Part model, mm, in its own coordinate system. A direction names the side the tool comes from. Round coordinates to 2 decimals unless told otherwise and drop trailing zeros. Write each loop counter-clockwise with the first axis right and the second up, starting at its lowest first coordinate (ties: lowest second). Pieces come first, ordered by that corner, then holes. Notation, with made-up numbers: (-20, -5) -> (-12, -5) arc R12 cw to (-12, 4) -> close; hole circle Ø10 at (-27, 2.5). An arc over 180 degrees is marked (long way). Return JSON: item names as keys, results as strings. Group by question number.
```python
from build123d import *

# Parameters (mm, degrees)
SKETCH1_W           = 366
SKETCH1_H           = 19
BOSS_EXTRUDE2_DEPTH = 19
SKETCH9_W           = 17
SKETCH9_H           = 17
CUT_EXTRUDE4_DEPTH  = 367.985013318
CUT_EXTRUDE6_DEPTH  = 339.005366679
SKETCH12_R          = 2
CUT_EXTRUDE7_DEPTH  = 339.005366679


with BuildPart() as part:
    # Sketch1 → Boss-Extrude2 (new body)
    with BuildSketch(Plane(origin=(0, 0, 0), x_dir=(1, 0, 0), z_dir=(0, 1, 0))):
        with Locations((-153.935643564, 9.5)):
            Rectangle(SKETCH1_W, SKETCH1_H)
    extrude(amount=BOSS_EXTRUDE2_DEPTH)

    # Sketch9 → Cut-Extrude4 (cut, through all)
    with BuildSketch(Plane(origin=(29.064356436, 0, 0), x_dir=(0, 0, -1), z_dir=(1, 0, 0))):
        with Locations((9.5, 9.5)):
            Rectangle(SKETCH9_W, SKETCH9_H)
    extrude(amount=-CUT_EXTRUDE4_DEPTH, mode=Mode.SUBTRACT)

    # Sketch11 → Cut-Extrude6 (cut, through all)
    with BuildSketch(Plane(origin=(0, 0, -19), x_dir=(-1, 0, 0), z_dir=(0, 0, -1))):
        Polygon((-29.064356436, 19), (-29.064356436, 0), (3.935643564, 0), align=None)
        Polygon((336.935643564, 19), (336.935643564, 0), (303.935643564, 0), align=None)
    extrude(amount=-CUT_EXTRUDE6_DEPTH, mode=Mode.SUBTRACT)

    # Sketch12 → Cut-Extrude7 (cut, through all)
    with BuildSketch(Plane.XY):
        with Locations((-153.935643564, 10)):
            Circle(SKETCH12_R)
    extrude(amount=-CUT_EXTRUDE7_DEPTH, mode=Mode.SUBTRACT)


solid = part.part
```
Item 1: Flat gauge pin, fed straight in: P1, Ø5, axis at y = 3, z = -8.5, coming from the +X side. Where does the tip first touch, or does it go through?
Item 2: Cut at B-B (x = -119.5). Write the cut outline in (y, z).
Item 3: Cut at A-A (z = -14.5). Write the cut outline in (x, y).
Item 4: Wall check: L1, parallel to Y at x = -9, z = -4.5; L2, parallel to Z at x = 12, y = 14; L3, parallel to Y at x = 5, z = -9.25. Give the ranges that are in metal, low to high.
Item 5: Two-plate mould, pull along Y, no slides. Class faces 1 (the face through (-156, 9, -19)), 2 (the face through (-151, 18, -9)), 3 (the face through (11.265, 8.752, -0.396)), 4 (the face through (-151, 9, -1)): released by +Y, released by -Y, zero draft, split by the parting line, or undercut.
Item 6: Which spindle directions (+Z, -Z, +X, -X, +Y, -Y) get a long thin tool onto all of the face, cutting with end or side? Do faces 5 (the face through (-319.136, 8.752, -0.396)), 6 (the face through (-151, 9, -18)). Say none if no direction does.
Checks:
{
 "1": {"P1": "stops at x = -2.2"},
 "2": {"outline": "(0, -19) -> (19, -19) -> (19, 0) -> (0, 0) -> close; hole (1, -18) -> (18, -18) -> (18, -1) -> (1, -1) -> close"},
 "3": {"outline": "(-336.94, 19) -> (-335.2, 18) -> (27.33, 18) -> (29.06, 19) -> close; (-305.67, 1) -> (-303.94, 0) -> (-3.94, 0) -> (-2.2, 1) -> close"},
 "4": {"L1": "y = 0 to 1, 18 to 19", "L2": "z = -19 to -18, -1 to 0", "L3": "y = 18 to 19"},
 "5": {"face 1": "zero draft", "face 2": "undercut", "face 3": "released by -Y", "face 4": "undercut"},
 "6": {"face 5": "+Z, -Z, -X, -Y", "face 6": "+X, -X"}
}
